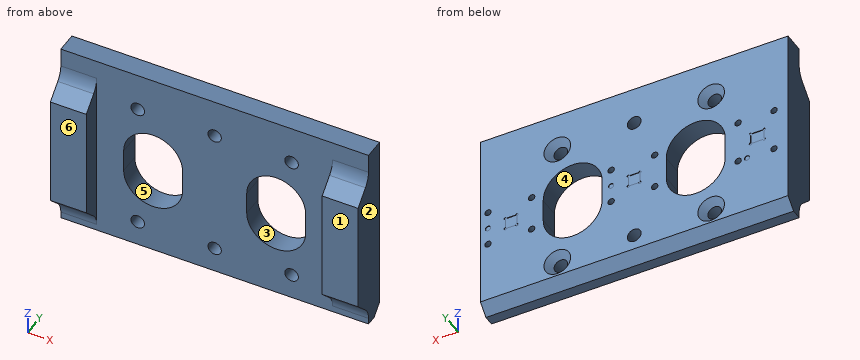
from build123d import *

# Parameters (mm, degrees)
SKETCH_5_W                  = 120
SKETCH_5_H                  = 75
EXTRUDE_2_DEPTH             = 8
SKETCH2_R                   = 1
CUT_EXTRUDE2_DEPTH          = 0.2
SKETCH3_R                   = 1
CUT_EXTRUDE3_DEPTH          = 0.2
M3X0_5_TAPPED_HOLE1_D       = 2.5
M3X0_5_TAPPED_HOLE1_DEPTH   = 5.5
M3X0_5_TAPPED_HOLE1_TIP     = 0.751075774
HOLE_WIZARD_M51_D           = 5.3
HOLE_WIZARD_M51_CSINK_D     = 10.4
HOLE_WIZARD_M51_CSINK_ANGLE = 90
SKETCH6_R                   = 2.6
CUT_EXTRUDE4_DEPTH          = 9
CUT_EXTRUDE4_TAPER          = -0.573055556
CUT_EXTRUDE_1_DEPTH         = 10
EXTRUDE_3_DEPTH             = 120
SKETCH_9_W                  = 92
SKETCH_9_H                  = 19.20799114
CUT_EXTRUDE_3_DEPTH         = 76
CHAMFER_1_SIZE              = 4


with BuildPart() as part:
    # Эскиз5 → Бобышка-Вытянуть2 (new body)
    with BuildSketch(Plane(origin=(0, 0, 0), x_dir=(1, 0, 0), z_dir=(0, 1, 0))):
        with Locations((60, -2.5)):
            Rectangle(SKETCH_5_W, SKETCH_5_H)
    extrude(amount=-EXTRUDE_2_DEPTH)

    # Sketch2 → Cut-Extrude2 (cut)
    with BuildSketch(Plane(origin=(0, 0, 0), x_dir=(1, 0, 0), z_dir=(0, 1, 0))):
        with Locations((117.027, -0.519)):
            Circle(SKETCH2_R)
        with Locations((69.027, -0.519)):
            Circle(SKETCH2_R)
        with BuildLine():
            Line((106.24, -2.26), (109.76, -2.26))
            ThreePointArc((109.76, -2.26), (110.613553391, -2.613553391), (110.26, -1.76))
            Line((110.26, -1.76), (110.26, 1.76))
            ThreePointArc((110.26, 1.76), (110.613553391, 2.613553391), (109.76, 2.26))
            Line((109.76, 2.26), (106.24, 2.26))
            ThreePointArc((106.24, 2.26), (105.386446609, 2.613553391), (105.74, 1.76))
            Line((105.74, 1.76), (105.74, -1.76))
            ThreePointArc((105.74, -1.76), (105.386446609, -2.613553391), (106.24, -2.26))
        make_face()
        with BuildLine():
            Line((58.24, -2.26), (61.76, -2.26))
            ThreePointArc((61.76, -2.26), (62.613553391, -2.613553391), (62.26, -1.76))
            Line((62.26, -1.76), (62.26, 1.76))
            ThreePointArc((62.26, 1.76), (62.613553391, 2.613553391), (61.76, 2.26))
            Line((61.76, 2.26), (58.24, 2.26))
            ThreePointArc((58.24, 2.26), (57.386446609, 2.613553391), (57.74, 1.76))
            Line((57.74, 1.76), (57.74, -1.76))
            ThreePointArc((57.74, -1.76), (57.386446609, -2.613553391), (58.24, -2.26))
        make_face()
    extrude(amount=-CUT_EXTRUDE2_DEPTH, mode=Mode.SUBTRACT)

    # Sketch3 → Cut-Extrude3 (cut)
    with BuildSketch(Plane(origin=(0, 0, 0), x_dir=(1, 0, 0), z_dir=(0, 1, 0))):
        with Locations((16, 8)):
            Circle(SKETCH3_R)
        with BuildLine():
            Line((9.86, -2.16), (14.14, -2.16))
            ThreePointArc((14.14, -2.16), (14.993553391, -2.513553391), (14.64, -1.66))
            Line((14.64, -1.66), (14.64, 1.66))
            ThreePointArc((14.64, 1.66), (14.993553391, 2.513553391), (14.14, 2.16))
            Line((14.14, 2.16), (9.86, 2.16))
            ThreePointArc((9.86, 2.16), (9.006446609, 2.513553391), (9.36, 1.66))
            Line((9.36, 1.66), (9.36, -1.66))
            ThreePointArc((9.36, -1.66), (9.006446609, -2.513553391), (9.86, -2.16))
        make_face()
    extrude(amount=-CUT_EXTRUDE3_DEPTH, mode=Mode.SUBTRACT)

    # M3x0.5 Tapped Hole1
    with Locations(Plane(origin=(0, 0, 0), x_dir=(1, 0, 0), z_dir=(0, 1, 0))):
        with Locations((5.5, 8), (19.5, 8), (19.5, -9), (5.5, -9), (52.027, 6.481), (69.027, 6.481), (69.027, -7.519), (52.027, -7.519), (100.027, 6.481), (117.027, 6.481), (117.027, -7.519), (100.027, -7.519)):
            Hole(M3X0_5_TAPPED_HOLE1_D / 2, depth=M3X0_5_TAPPED_HOLE1_DEPTH)
            with Locations((0, 0, -(M3X0_5_TAPPED_HOLE1_DEPTH + M3X0_5_TAPPED_HOLE1_TIP / 2))):  # 118° drill point
                Cone(0, M3X0_5_TAPPED_HOLE1_D / 2, M3X0_5_TAPPED_HOLE1_TIP, mode=Mode.SUBTRACT)

    # Зенковка для  винта с плоской головкой M51 (through all)
    with Locations(Plane(origin=(0, 0, 0), x_dir=(1, 0, 0), z_dir=(0, 1, 0))):
        with Locations((30, 25), (90, 25), (90, -25), (30, -25)):
            CounterSinkHole(HOLE_WIZARD_M51_D / 2, HOLE_WIZARD_M51_CSINK_D / 2, counter_sink_angle=HOLE_WIZARD_M51_CSINK_ANGLE)

    # Sketch6 → Cut-Extrude4 (cut, through all)
    with BuildSketch(Plane.XZ.offset(8)):
        with Locations((60, -25)):
            Circle(SKETCH6_R)
        with Locations((60, 25)):
            Circle(SKETCH6_R)
    extrude(amount=-CUT_EXTRUDE4_DEPTH, taper=CUT_EXTRUDE4_TAPER, mode=Mode.SUBTRACT)

    # Эскиз7 → Вырез-Вытянуть1 (cut)
    with BuildSketch(Plane(origin=(0, 0, 0), x_dir=(1, 0, 0), z_dir=(0, 1, 0))):
        with BuildLine():
            Line((47.5, 4.354177178), (47.5, -4.354177178))
            ThreePointArc((47.5, -4.354177178), (36, -15.854177178), (24.5, -4.354177178))
            Line((24.5, -4.354177178), (24.5, 4.354177178))
            ThreePointArc((24.5, 4.354177178), (36, 15.854177178), (47.5, 4.354177178))
        make_face()
        with BuildLine():
            Line((95.5, 4.354177178), (95.5, -4.354177178))
            ThreePointArc((95.5, -4.354177178), (84, -15.854177178), (72.5, -4.354177178))
            Line((72.5, -4.354177178), (72.5, 4.354177178))
            ThreePointArc((72.5, 4.354177178), (84, 15.854177178), (95.5, 4.354177178))
        make_face()
    extrude(amount=-CUT_EXTRUDE_1_DEPTH, mode=Mode.SUBTRACT)

    # Эскиз8 → Бобышка-Вытянуть3 (add, through all)
    with BuildSketch(Plane(origin=(120, 0, 0), x_dir=(0, 0, -1), z_dir=(1, 0, 0))):
        with BuildLine():
            Line((-21.893398282, -15.5), (21.893398282, -15.5))
            Line((21.893398282, -15.5), (27.196699141, -10.196699141))
            ThreePointArc((27.196699141, -10.196699141), (29.629874257, -8.570903506), (32.5, -8))
            Line((32.5, -8), (-32.5, -8))
            ThreePointArc((-32.5, -8), (-29.629874257, -8.570903506), (-27.196699141, -10.196699141))
            Line((-27.196699141, -10.196699141), (-21.893398282, -15.5))
        make_face()
    extrude(amount=-EXTRUDE_3_DEPTH)

    # Эскиз9 → Вырез-Вытянуть3 (cut, through all)
    with BuildSketch(Plane.XY.offset(40)):
        with Locations((60, -17.60399557)):
            Rectangle(SKETCH_9_W, SKETCH_9_H)
    extrude(amount=-CUT_EXTRUDE_3_DEPTH, mode=Mode.SUBTRACT)

    # Фаска1
    chamfer_1_edges = [part.edges().sort_by_distance(p)[0] for p in [
        (60, 0, -35),
    ]]
    chamfer(chamfer_1_edges, length=CHAMFER_1_SIZE)


solid = part.part
Geometry: final body of the model. Coordinates: model frame, mm. Face numbers are marked on the shaded views. A direction names the side the tool comes from. Round coordinates to 2 decimals unless told otherwise and drop trailing zeros. Loops run counter-clockwise (first coordinate to the right, second up) from the corner with the lowest first, then second, coordinate; pieces in that order, holes last. Notation, with made-up numbers: (-31, -9.5) - (1, -9.5) arc R23 cw to (1, 4.5) - close; hole circle Ø7 at (2, -31). An arc over 180 degrees is marked (long way). Write each question's results on one line, items separated by ' | '. Start each with the question number.
1) Cut plane A-A on x = 30. Return loops of the section in (y, z).
2) Cut plane C-C on x = 75. Return loops of the section in (y, z).
3) Mould query, pull axis X, two halves, no side actions, for the marked faces 1, 2, 3 and 4. Classes: released by +X, released by -X, zero draft, split by the parting line, or undercut.
4) Line query: probe 1 along X at (y, z) = (-10, -15.5); probe 2 along X at (y, z) = (-6.35, -25); probe 3 along Y at (x, z) = (82, 28). Output: solid intervals per line, ascending. Write a range as [from, to].
5) Cut plane B-B on z = 13. Return loops of the section in (x, y), then the cut area to 3 significant figures.
6) Cut plane D-D on x = 12.5. Return loops of the section in (y, z).
7) Access query for the marked faces 5 and 6. Directions: +Z, -Z, +X, -X, +Y, -Y. A direction counts if a zero-diameter tool reaches every point of the face in a straight line with its end or side. Return the directions, or none.
8) First-contact query: P1, Ø3, axis at x = 117.027, z = 7.519, coming from the +Y side; P2, Ø2, axis at x = 31.5, z = -21.5, coming from the +Y side; P3, Ø7, axis at x = 90, z = -25, coming from the -Y side; P4, Ø1.6, axis at x = 117.027, z = 0.519, coming from the +Y side. Flat tips, straight axial feed; report the tip coordinate or a pass-through.
Verdict:
1) outline: (-8, -35) - (-4, -35) - (0, -31) - (0, -30.2) - (-2.55, -27.65) - (-8, -27.65) - close; (-8, -22.35) - (-2.55, -22.35) - (0, -19.8) - (0, -14.16) - (-8, -14.16) - close; (-8, 14.16) - (0, 14.16) - (0, 19.8) - (-2.55, 22.35) - (-8, 22.35) - close; (-8, 27.65) - (-2.55, 27.65) - (0, 30.2) - (0, 40) - (-8, 40) - close
2) outline: (-8, -35) - (-4, -35) - (0, -31) - (0, -11.51) - (-8, -11.51) - close; (-8, 11.51) - (0, 11.51) - (0, 40) - (-8, 40) - close
3) face 1: zero draft | face 2: released by +X | face 3: undercut | face 4: undercut
4) probe 1: x = [0, 14], [106, 120] | probe 2: x = [0, 27.35], [32.65, 57.38], [62.62, 87.35], [92.65, 120] | probe 3: y = [-8, 0]
5) outline: (0, -15.5) - (14, -15.5) - (14, -8) - (28.42, -8) - (28.42, 0) - (0, 0) - close; (43.58, -8) - (76.42, -8) - (76.42, 0) - (43.58, 0) - close; (91.58, -8) - (106, -8) - (106, -15.5) - (120, -15.5) - (120, 0) - (91.58, 0) - close | area: 927 mm2
6) outline: (-15.5, -21.89) - (-10.2, -27.2) arc R7.5 cw to (-8, -32.5) - (-8, -35) - (-4, -35) - (0, -31) - (0, -2.16) - (-0.2, -2.16) - (-0.2, 2.16) - (0, 2.16) - (0, 40) - (-8, 40) - (-8, 32.5) arc R7.5 cw to (-10.2, 27.2) - (-15.5, 21.89) - close
7) face 5: +Y, -Y | face 6: +Z, -Z, +X, -X, -Y
8) P1: stops at y = 0 | P2: stops at y = -0.39 | P3: stops at y = -8 | P4: stops at y = -0.2
